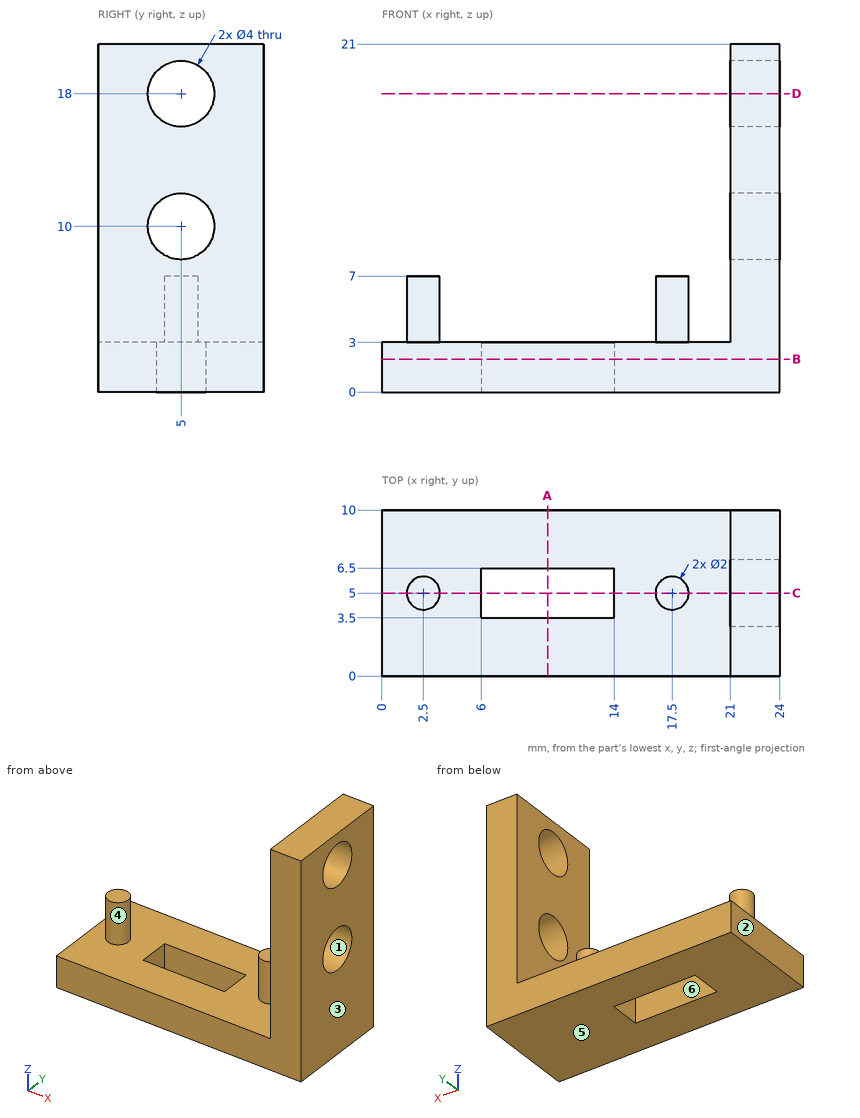
For this review, use the dimensioned drawing (mm, ordinates from the lowest corner) and the shaded views. A direction names the side the tool comes from. Give positions to 0.01 mm unless a question says otherwise; leave off trailing zeros. Order: outer loops, then holes, each group sorted by start corner. A loop starts at its lowest first (then second) coordinate and runs counter-clockwise, first axis right, second up.
1. To check wall thickness, follow L1, parallel to Z at x = 22.65, y = 5; L2, parallel to Z at x = 7.5, y = 9.5; L3, parallel to X at y = 8.75, z = 16. State the ranges of each line that lie inside material, in increasing order.
Solution:
L1: z = 0 to 8, 12 to 16, 20 to 21
L2: z = 0 to 3
L3: x = 21 to 24
2. Tool access review of the marked faces 5 and 6: name each direction out of +Z, -Z, +X, -X, +Y, -Y from which nothing blocks a thin tool from reaching the whole face with its end or side.
Solution:
face 5: -Z, +X, -X, +Y, -Y
face 6: +Z, -Z
3. Mouldability with a two-part tool opening along X and no side actions: class the marked faces 1, 2, 3 and 4 as +X half, -X half, draft (parallel to the pull), parting line (faces both ways), or undercut.
Solution:
face 1: draft
face 2: -X half
face 3: +X half
face 4: undercut
4. Add section B-B, the plane z = 2. State the section outline as (x, y) points, then the cut area to 3 significant figures.
Solution:
outline: (0, 0) - (24, 0) - (24, 10) - (0, 10) - close; hole (6, 3.5) - (14, 3.5) - (14, 6.5) - (6, 6.5) - close
area: 216 mm2
5. For pin 1 Ø1 at (x, y) = (2.5, 4.5) entering from +Z; pin 2 Ø3 at (y, z) = (5, 12) entering from -X; pin 3 Ø5 at (x, y) = (9, 4.5) entering from +Z, all flat-tipped, find the tip position at first contact; note any pin that passes through.
Solution:
pin 1: stops at z = 7
pin 2: stops at x = 21
pin 3: stops at z = 3
6. Add section D-D, the plane z = 18. State the section outline as (x, y) points.
Solution:
outline: (21, 0) - (24, 0) - (24, 3) - (21, 3) - close; (21, 7) - (24, 7) - (24, 10) - (21, 10) - close
7. Add section A-A, the plane x = 10. State the section outline as (y, z) points, then the cut area to 3 significant figures.
Solution:
outline: (0, 0) - (3.5, 0) - (3.5, 3) - (0, 3) - close; (6.5, 0) - (10, 0) - (10, 3) - (6.5, 3) - close
area: 21.0 mm2
8. Add section C-C, the plane y = 5. State the section outline as (x, z) points, then the cut area to 3 significant figures.
Solution:
outline: (0, 0) - (6, 0) - (6, 3) - (3.5, 3) - (3.5, 7) - (1.5, 7) - (1.5, 3) - (0, 3) - close; (14, 0) - (24, 0) - (24, 8) - (21, 8) - (21, 3) - (18.5, 3) - (18.5, 7) - (16.5, 7) - (16.5, 3) - (14, 3) - close; (21, 12) - (24, 12) - (24, 16) - (21, 16) - close; (21, 20) - (24, 20) - (24, 21) - (21, 21) - close
area: 94.0 mm2
